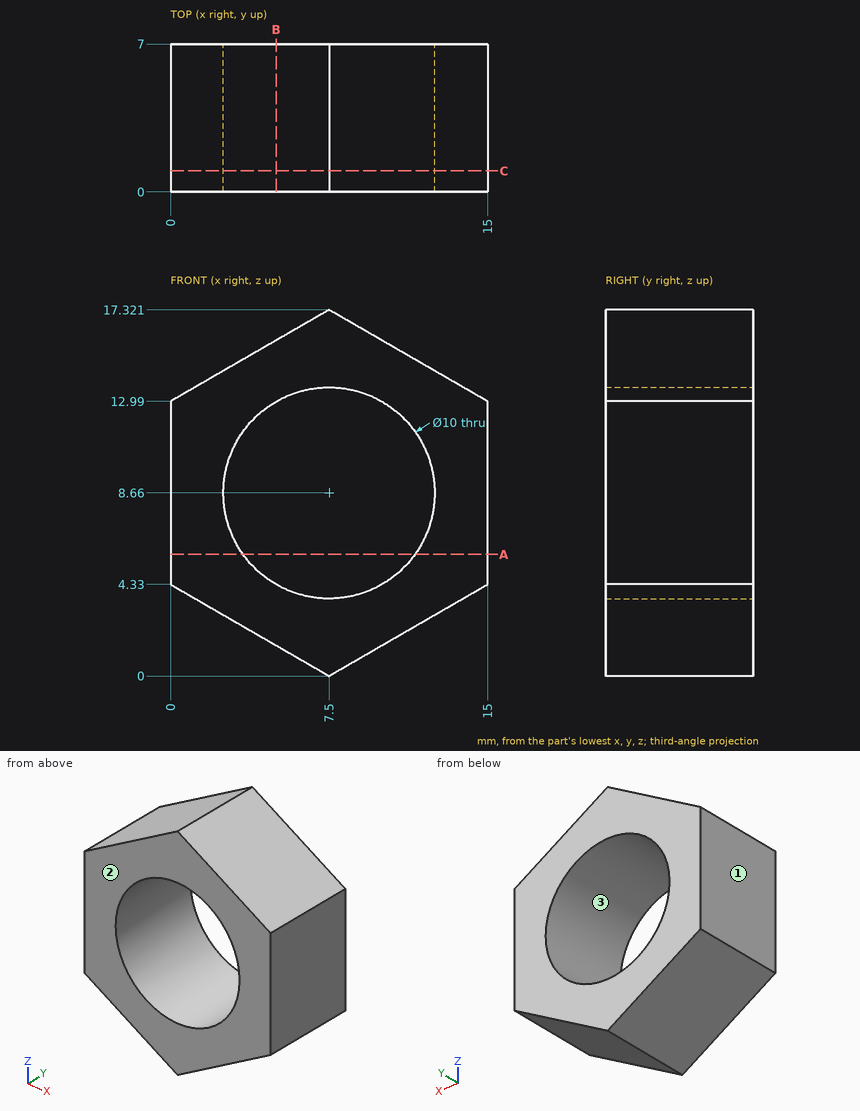
Job drawing, mm, ordinate dimensions from the low corner. One solid piece. Give positions to 0.01 mm unless a question says otherwise; leave off trailing zeros. Loops run counter-clockwise (first coordinate to the right, second up) from the corner with the lowest first, then second, coordinate; pieces in that order, holes last.
Item 1: Slice it at A-A, the plane z = 5.75. List the corners of the cut face in (x, y) (1 decimal).
Answers follow:
outline: (0, 0) - (3.4, 0) - (3.4, 7) - (0, 7) - close; (11.6, 0) - (15, 0) - (15, 7) - (11.6, 7) - close
Item 2: Slice it at B-B, the plane x = 5. List the corners of the cut face in (y, z).
Answers follow:
outline: (0, 1.44) - (7, 1.44) - (7, 4.33) - (0, 4.33) - close; (0, 12.99) - (7, 12.99) - (7, 15.88) - (0, 15.88) - close
Item 3: Slice it at C-C, the plane y = 1. List the corners of the cut face in (x, z).
Answers follow:
outline: (0, 4.33) - (7.5, 0) - (15, 4.33) - (15, 12.99) - (7.5, 17.32) - (0, 12.99) - close; hole circle Ø10 at (7.5, 8.66)
Item 4: Pull direction X, two halves, no side cores. Call the marked faces 1, 2 and 3: released by +X, released by -X, zero draft, split by the parting line, or undercut.
Answers follow:
face 1: released by -X
face 2: zero draft
face 3: undercut
Item 5: Flat gauge pins, fed straight in: pin 1 (1 mm diameter, centred on x = 6, y = 2.5, fed in from +Z); pin 2 (3 mm diameter, centred on x = 11.5, y = 2.5, fed in from -Z). Where does each tip first touch, or does it go through?
Answers follow:
pin 1: stops at z = 16.74
pin 2: stops at z = 1.44
Item 6: Drill centre lines: line 1 (X direction, y = 1.75, z = 12.5) (1 decimal); line 2 (X direction, y = 0.5, z = 5.5) (1 decimal); line 3 (Z direction, x = 11.5, y = 3.25). Where is each one in solid material? Low to high.
Answers follow:
line 1: x = 0 to 4.3, 10.7 to 15
line 2: x = 0 to 3.6, 11.4 to 15
line 3: z = 2.31 to 5.66, 11.66 to 15.01
